Here's the drawing with two shaded views (mm, measured from the low corner). I have some questions. A direction names the side the tool comes from. Coordinates: 2 decimals unless noted, no trailing zeros. Order: outer loops, then holes, each group sorted by start corner. A loop starts at its lowest first (then second) coordinate and runs counter-clockwise, first axis right, second up. Notation, with made-up numbers: (64.25, 81.25) - (113.25, 81.25) arc R23 ccw to (113.25, 101.25) - close; hole circle Ø9 at (-2, 7). An arc over 180 degrees is marked (long way). Answer as a JSON object with one key per item and string values. Group by question number.
(1) Imagine slicing it at A-A, the plane x = 15. Write out the boundary of the cut face in (y, z).
(2) Will these pins go through, and if not, where does the flat tip stop? P1, Ø9.5, axis at x = 77, z = 7, coming from the +Y side; P2, Ø3, axis at x = 72, y = 17, coming from the -Z side; P3, Ø8, axis at x = 14.5, y = 62.5, coming from the +Z side.
(3) Imagine slicing it at C-C, the plane y = 34.5. Write out the boundary of the cut face in (x, z) (3 decimals).
(4) Imagine slicing it at B-B, the plane z = 9. Write out the boundary of the cut face in (x, y) (1 decimal), and give its area (3 significant figures).
(5) Which directions (+Z, -Z, +X, -X, +Y, -Y) give clear straight access to the entire face, cutting with the end or side of a thin tool? Please do the marked faces 1, 2, 3 and 4.
(6) Imagine slicing it at D-D, the plane x = 49. Write out the boundary of the cut face in (y, z).
(7) Please list where these lines run through material, in increasing order: probe 1 along Y at (x, z) = (16.25, 10); probe 2 along Z at (x, y) = (19, 65); probe 3 along Y at (x, z) = (34, 16.5).
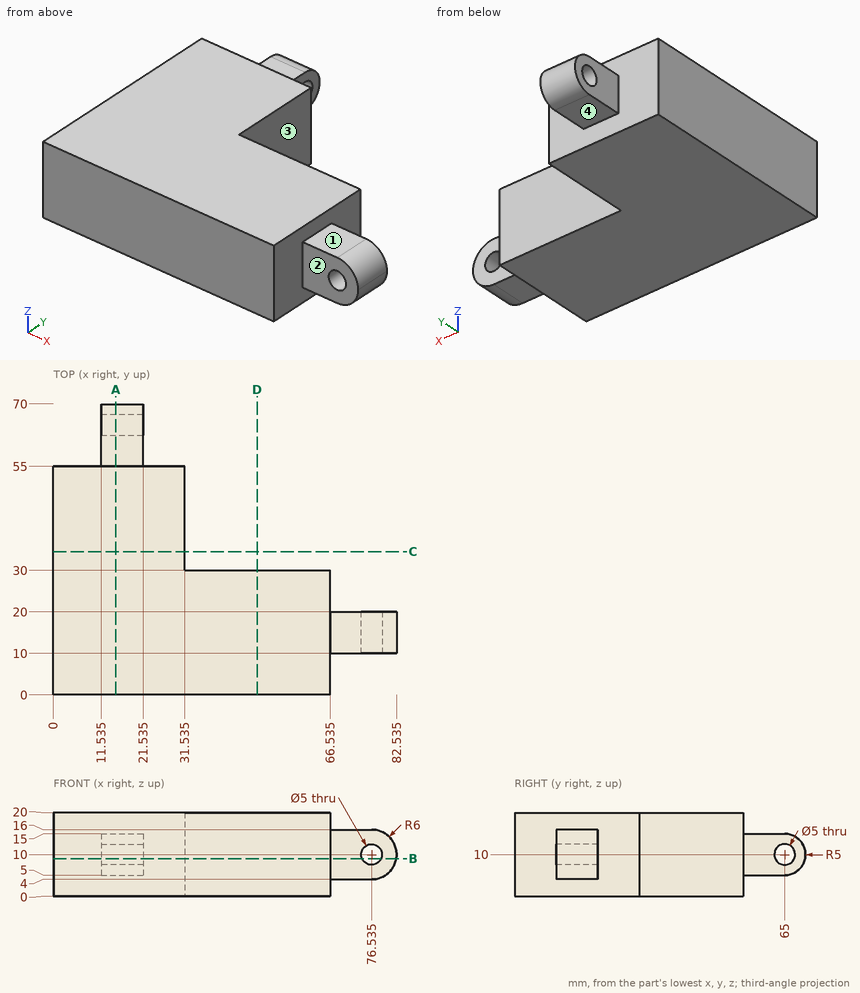
Result set:
{
 "1": {"outline": "(0, 0) - (55, 0) - (55, 5) - (65, 5) arc R5 ccw to (65, 15) - (55, 15) - (55, 20) - (0, 20) - close; hole circle Ø5 at (65, 10)"},
 "2": {"P1": "stops at y = 20", "P2": "stops at z = 4", "P3": "stops at z = 15"},
 "3": {"outline": "(0, 0) - (31.535, 0) - (31.535, 20) - (0, 20) - close"},
 "4": {"outline": "(0, 0) - (66.5, 0) - (66.5, 10) - (74.2, 10) - (74.2, 20) - (66.5, 20) - (66.5, 30) - (31.5, 30) - (31.5, 55) - (21.5, 55) - (21.5, 62.7) - (11.5, 62.7) - (11.5, 55) - (0, 55) - close; (11.5, 67.3) - (21.5, 67.3) - (21.5, 69.9) - (11.5, 69.9) - close; (78.8, 10) - (82.5, 10) - (82.5, 20) - (78.8, 20) - close", "area": "3,000 mm^2"},
 "5": {"face 1": "+Z, +X, +Y, -Y", "face 2": "+Z, -Z, +X, -Y", "face 3": "+Z, -Z, +X, +Y", "face 4": "-Z, +X, -X, +Y"},
 "6": {"outline": "(0, 0) - (30, 0) - (30, 20) - (0, 20) - close"},
 "7": {"probe 1": "y = 0 to 62.5, 67.5 to 70", "probe 2": "z = 5 to 7.5, 12.5 to 15", "probe 3": "y = 0 to 30"}
}
